Autodesk Inventor part; units mm, degrees
ref_plane "YZ Plane" through (0, 0, 0) normal (1, 0, 0) x (0, 1, 0)
ref_plane "XZ Plane" through (0, 0, 0) normal (0, 1, 0) x (-1, 0, 0)
ref_plane "XY Plane" through (0, 0, 0) normal (0, 0, 1) x (1, 0, 0)
sketch "Эскиз1" plane through (0, 0, 0) normal (0, 1, 0) x (-1, 0, 0)
  line L0 (0, 0) -> (54.5, 0)
  line L1 (54.5, 0) -> (54.5, -54.5)
  line L2 (54.5, -54.5) -> (0, -54.5)
  line L3 (0, -54.5) -> (0, 0)
  dimension "d0" = 54.5
  dimension "d1" = 54.5
extrude "Выдавливание1" add sketch "Эскиз1" along normal blind 4
fillet "Сопряжение1" radius 3 4 edges at (0, 2, 0) (0, 2, -54.5) (-54.5, 2, -54.5) (-54.5, 2, 0)
sketch "Эскиз2" plane through (0, 0, 0) normal (0, -1, 0) x (1, 0, 0)
  arc A0 (-54.5, -51.5) -> (-51.5, -54.5) centre (-51.5, -51.5) ccw
  line L0 (-54.5, -51.5) -> (-54.5, -3)
  line L1 (-54.5, -27.25) -> (0, -27.25) construction
  line L2 (0, -3) -> (0, -51.5)
  line L3 (-3, -54.5) -> (-51.5, -54.5)
  line L4 (-27.25, -54.5) -> (-27.25, 0) construction
  line L5 (-51.5, 0) -> (-3, 0)
  line L6 (-54.5, -51.5) -> (-54.5, -3)
  circle A1 centre (-49.25, -49.25) radius 3
  circle A2 centre (-49.25, -5.25) radius 3
  circle A3 centre (-5.25, -49.25) radius 3
  circle A4 centre (-5.25, -5.25) radius 3
  point P0 (0, 0)
  dimension "d13" = 6
  dimension "d34" = 44
  dimension "d35" = 44
extrude "Выдавливание2" cut sketch "Эскиз2" against normal blind 2
sketch "Эскиз3" plane through (0, 2, 0) normal (0, -1, 0) x (1, 0, 0)
  circle A0 centre (-49.25, -49.25) radius 1.75
  line L0 (-54.5, -51.5) -> (-54.5, -3)
  line L1 (-54.5, -27.25) -> (0, -27.25) construction
  line L2 (0, -3) -> (0, -51.5)
  line L3 (-3, -54.5) -> (-51.5, -54.5)
  line L4 (-27.25, -54.5) -> (-27.25, 0) construction
  line L5 (-51.5, 0) -> (-3, 0)
  circle A1 centre (-49.25, -5.25) radius 1.75
  circle A2 centre (-5.25, -49.25) radius 1.75
  circle A3 centre (-5.25, -5.25) radius 1.75
  circle A4 centre (-49.25, -49.25) radius 3 construction
  circle A5 centre (-49.25, -49.25) radius 3
  point P0 (0, 0)
  point P1 (-45.0293, -48.6853)
  point P2 (-51.4707, -47.8147)
  dimension "d9" = 3.5
extrude "Выдавливание3" cut sketch "Эскиз3" against normal blind 2 contours A0 | A1 | A2 | A3
sketch "Эскиз4" plane through (0, 4, 0) normal (0, 1, 0) x (1, 0, 0)
  line L0 (-54.5, 51.5) -> (-54.5, 3)
  line L1 (0, 3) -> (0, 51.5) construction
  line L2 (-51.5, 0) -> (-3, 0)
  line L3 (-3, 54.5) -> (-51.5, 54.5)
  line L4 (-49.5, 14.5) -> (0, 14.5) construction
  line L5 (0, 14.5) -> (0, 40) construction
  line L6 (0, 40) -> (-49.5, 40) construction
  line L7 (-49.5, 40) -> (-49.5, 14.5) construction
  line L8 (-46.25, 16.75) -> (-3.25, 16.75) construction
  line L9 (-3.25, 16.75) -> (-3.25, 37.75) construction
  line L10 (-3.25, 37.75) -> (-46.25, 37.75) construction
  line L11 (-46.25, 37.75) -> (-46.25, 16.75) construction
  line L12 (-24.75, 14.5) -> (-24.75, 40) construction
  line L13 (0, 27.25) -> (-24.75, 27.25) construction
  line L14 (-24.75, 16.75) -> (-24.75, 37.75) construction
  line L15 (-3.25, 27.25) -> (-24.75, 27.25) construction
  circle A0 centre (-46.25, 16.75) radius 1.5
  circle A1 centre (-46.25, 37.75) radius 1.5
  circle A2 centre (-3.25, 37.75) radius 1.5
  circle A3 centre (-3.25, 16.75) radius 1.5
  line L16 (-27.25, 27.25) -> (-21.7344, 27.25) construction
  point P0 (0, 0)
  dimension "d17" = 49.5
  dimension "d18" = 25.5
  dimension "d19" = 43
  dimension "d20" = 21
  dimension "d21" = 3
  dimension "d22" = 3
  dimension "d23" = 3
  dimension "d24" = 3
  dimension "d36" = 2.25
  dimension "d37" = 3.25
  dimension "d40" = 3.25
  dimension "d41" = 2.25
  dimension "d42" = 2.25
  dimension "d43" = 3.25
  dimension "d44" = 3.25
  dimension "d45" = 2.25
extrude "Выдавливание4" cut sketch "Эскиз4" against normal blind 4
sketch "Эскиз5" plane through (0, 0, 0) normal (0, -1, 0) x (1, 0, 0)
  circle A0 centre (-3.25, -16.75) radius 1.5
  circle A1 centre (-3.25, -16.75) radius 2.25 construction
  line L0 (-1, -16.75) -> (-2.125, -18.6986)
  line L1 (-2.125, -18.6986) -> (-4.375, -18.6986)
  line L2 (-4.375, -18.6986) -> (-5.5, -16.75)
  line L3 (-5.5, -16.75) -> (-4.375, -14.8014)
  line L4 (-4.375, -14.8014) -> (-2.125, -14.8014)
  line L5 (-2.125, -14.8014) -> (-1, -16.75)
  circle A2 centre (-3.25, -37.75) radius 1.5
  circle A3 centre (-3.25, -37.75) radius 1.5
  circle A4 centre (-46.25, -37.75) radius 1.5
  circle A5 centre (-46.25, -37.75) radius 1.5
  circle A6 centre (-46.25, -16.75) radius 1.5
  circle A7 centre (-46.25, -16.75) radius 1.5
  line L6 (-1, -37.75) -> (-2.125, -39.6986)
  line L7 (-2.125, -39.6986) -> (-4.375, -39.6986)
  line L8 (-4.375, -39.6986) -> (-5.5, -37.75)
  line L9 (-5.5, -37.75) -> (-4.375, -35.8014)
  line L10 (-4.375, -35.8014) -> (-2.125, -35.8014)
  line L11 (-2.125, -35.8014) -> (-1, -37.75)
  line L12 (-44, -37.75) -> (-45.125, -39.6986)
  line L13 (-45.125, -39.6986) -> (-47.375, -39.6986)
  line L14 (-47.375, -39.6986) -> (-48.5, -37.75)
  line L15 (-48.5, -37.75) -> (-47.375, -35.8014)
  line L16 (-47.375, -35.8014) -> (-45.125, -35.8014)
  line L17 (-45.125, -35.8014) -> (-44, -37.75)
  line L18 (-44, -16.75) -> (-45.125, -18.6986)
  line L19 (-45.125, -18.6986) -> (-47.375, -18.6986)
  line L20 (-47.375, -18.6986) -> (-48.5, -16.75)
  line L21 (-48.5, -16.75) -> (-47.375, -14.8014)
  line L22 (-47.375, -14.8014) -> (-45.125, -14.8014)
  line L23 (-45.125, -14.8014) -> (-44, -16.75)
  line L24 (-44, -16.75) -> (-48.5, -16.75) construction
  line L25 (-44, -37.75) -> (-48.5, -37.75) construction
  line L26 (-1, -37.75) -> (-5.5, -37.75) construction
  line L27 (-1, -16.75) -> (-5.5, -16.75) construction
  point P0 (0, 0)
  dimension "d27" = 4.5
extrude "Выдавливание5" cut sketch "Эскиз5" against normal blind 2 contours A0 | L0 L1 L2 L3 L4 L5 | A2 | A4 | A6 | L6 L7 L8 L9 L10 L11 | L12 L13 L14 L15 L16 L17 | L18 L19 L20 L21 L22 L23
sketch "Эскиз6" plane through (0, 0, 0) normal (0, -1, 0) x (1, 0, 0)
  circle A0 centre (-2.5, -33.5) radius 1.25
  line L0 (-2.5, -33.5) -> (-2.5, -21) construction
  circle A1 centre (-2.5, -21) radius 1.25
  line L1 (0, -3) -> (0, -51.5)
  line L2 (0, -3) -> (0, -51.5)
  line L3 (0, -27.25) -> (-19.5358, -27.25) construction
  point P0 (0, 0)
  point P1 (-2.5, -27.25)
  dimension "d46" = 2.5
  dimension "d47" = 12.5
  dimension "d48" = 2.5
  dimension "d49" = 2.5
extrude "Выдавливание6" cut sketch "Эскиз6" against normal blind 4
equation "\"d0\" = d1"
equation "\"d22\" = d21"
equation "\"d23\" = d21"
equation "\"d24\" = d21"
equation "\"d36\" = d42"
equation "\"d37\" = d43"
equation "\"d40\" = d43"
equation "\"d41\" = d42"
equation "\"d44\" = d43"
equation "\"d45\" = d42"
properties part number "bottom"
Here's how the part is built. I have some questions about the finished solid (model axes, mm). A direction names the side the tool comes from. Coordinates: 2 decimals unless noted, no trailing zeros. Order: outer loops, then holes, each group sorted by start corner. A loop starts at its lowest first (then second) coordinate and runs counter-clockwise, first axis right, second up.
Item 1: If we section it at C-C, the plane y = 3.35: Give the number of separate pieces and of enclosed holes in the cut face, then the cut area to 3 significant figures.
Response values:
separate pieces: 1
enclosed holes: 10
area: 2,890 mm2
Item 2: If we section it at D-D, the plane x = -50: List the corners of the cut face in (y, z) for me, then the cut area to 3 significant figures.
Response values:
outline: (0, -54.5) - (4, -54.5) - (4, -50.83) - (2, -50.83) - (2, -52.15) - (0, -52.15) - close; (0, -46.35) - (2, -46.35) - (2, -47.67) - (4, -47.67) - (4, -6.83) - (2, -6.83) - (2, -8.15) - (0, -8.15) - close; (0, -2.35) - (2, -2.35) - (2, -3.67) - (4, -3.67) - (4, 0) - (0, 0) - close
area: 182 mm2
Item 3: If we section it at B-B, the plane z = -49.25: List the corners of the cut face in (x, y) for me.
Response values:
outline: (-54.5, 0) - (-52.25, 0) - (-52.25, 2) - (-51, 2) - (-51, 4) - (-54.5, 4) - close; (-47.5, 2) - (-46.25, 2) - (-46.25, 0) - (-8.25, 0) - (-8.25, 2) - (-7, 2) - (-7, 4) - (-47.5, 4) - close; (-3.5, 2) - (-2.25, 2) - (-2.25, 0) - (0, 0) - (0, 4) - (-3.5, 4) - close
Item 4: I'm going to push a flat-ended pin straight in: pin 1 Ø1.2 at (x, z) = (-45.5, -37) entering from -Y. Where does the tip first touch, or does it pass through?
Response values:
pin 1: stops at y = 2
Item 5: Thinking about a two-plate mould opening in X: for faces 3 (the face through (-0.9, 2.03, -0.86)), 4 (the face through (-44.555, 0.986, -17.711)), 5 (the face through (-28, 2, -54.5)), which applies, pulls with the +X half, pulls with the -X half, needs draft (parallel to the pull), parting line crosses it, or undercut?
Response values:
face 3: pulls with the +X half
face 4: undercut
face 5: needs draft
Item 6: If we section it at A-A, the plane z = -21: List the corners of the cut face in (x, y) for me.
Response values:
outline: (-54.5, 0) - (-3.75, 0) - (-3.75, 4) - (-54.5, 4) - close; (-1.25, 0) - (0, 0) - (0, 4) - (-1.25, 4) - close
Item 7: I need wall thicknesses on probe 1 along Z at (x, y) = (-49.5, 1.3); probe 2 along Z at (x, y) = (-5.25, 3.3); probe 3 along X at (y, z) = (2.75, -37.75). Which ranges of each line are inside material? Lowest first, please.
Response values:
probe 1: z = -54.5 to -52.24, -46.26 to -8.24, -2.26 to 0
probe 2: z = -54.5 to -51, -47.5 to -7, -3.5 to 0
probe 3: x = -54.5 to -47.75, -44.75 to -4.75, -1.75 to 0
Item 8: Which directions (+Z, -Z, +X, -X, +Y, -Y) give clear straight access to the entire face, cutting with the end or side of a thin tool? Please do faces 1 (the face through (-48, 2, -7)), 2 (the face through (-53.64, 2.03, -0.9)).
Response values:
face 1: -Y
face 2: +Z, -X, +Y, -Y
